Part model, mm, in its own coordinate system. A direction names the side the tool comes from. Give positions to 0.01 mm unless a question says otherwise; leave off trailing zeros. Loops run counter-clockwise (first coordinate to the right, second up) from the corner with the lowest first, then second, coordinate; pieces in that order, holes last. Notation, with made-up numbers: (34, 40) -> (40, 40) arc R21 cw to (40, 45) -> close; hole circle Ø1 at (31, -15). An arc over 180 degrees is marked (long way). One line per question, with ' | ' between items.
```python
from build123d import *

# Parameters (mm, degrees)
SKETCH1_W          = 42
SKETCH1_H          = 42
BASE_FLANGE1_DEPTH = 4
SKETCH4_R          = 2.25
TAB1_DEPTH         = 4
SKETCH5_R          = 12
SKETCH5_R_2        = 2
CUT_EXTRUDE1_DEPTH = 40.73977856


# Sheet-metal steps are written as plain solids
with BuildPart() as part:
    # Sketch1 → Base-Flange1 (new body)
    with BuildSketch(Plane(origin=(0, 0, 0), x_dir=(1, 0, 0), z_dir=(0, 1, 0))):
        Rectangle(SKETCH1_W, SKETCH1_H)
    extrude(amount=-BASE_FLANGE1_DEPTH)

    # Sketch4 → Tab1 (add)
    # profile 1 of 2: a face of its own
    with BuildSketch(Plane(origin=(0, 0, 0), x_dir=(1, 0, 0), z_dir=(0, 1, 0))):
        with BuildLine():
            Line((-9, 27.5), (-9, -27.5))
            ThreePointArc((-9, -27.5), (-15, -33.5), (-21, -27.5))
            Line((-21, -27.5), (-21, 27.5))
            ThreePointArc((-21, 27.5), (-15, 33.5), (-9, 27.5))
        make_face()
        with Locations(Location((-15, 27.5, 0), (0, 0, 270))):
            Circle(SKETCH4_R, mode=Mode.SUBTRACT)
        with Locations(Location((-15, -27.5, 0), (0, 0, 270))):
            Circle(SKETCH4_R, mode=Mode.SUBTRACT)
    # profile 2 of 2: a face of its own
    with BuildSketch(Plane(origin=(0, 0, 0), x_dir=(1, 0, 0), z_dir=(0, 1, 0))):
        with BuildLine():
            Line((21, 27.5), (21, -27.5))
            ThreePointArc((21, -27.5), (15, -33.5), (9, -27.5))
            Line((9, -27.5), (9, 27.5))
            ThreePointArc((9, 27.5), (15, 33.5), (21, 27.5))
        make_face()
        with Locations(Location((15, 27.5, 0), (0, 0, 270))):
            Circle(SKETCH4_R, mode=Mode.SUBTRACT)
        with Locations(Location((15, -27.5, 0), (0, 0, 270))):
            Circle(SKETCH4_R, mode=Mode.SUBTRACT)
    extrude(amount=-TAB1_DEPTH)

    # Sketch5 → Cut-Extrude1 (cut, through all)
    with BuildSketch(Plane(origin=(0, 0, 0), x_dir=(1, 0, 0), z_dir=(0, 1, 0))):
        with Locations(Location((0, 0, 0), (0, 0, 270))):
            Circle(SKETCH5_R)
        with Locations(Location((15.5, 15.5, 0), (0, 0, 270))):
            Circle(SKETCH5_R_2)
        with Locations(Location((15.5, -15.5, 0), (0, 0, 270))):
            Circle(SKETCH5_R_2)
        with Locations(Location((-15.5, -15.5, 0), (0, 0, 270))):
            Circle(SKETCH5_R_2)
        with Locations(Location((-15.5, 15.5, 0), (0, 0, 270))):
            Circle(SKETCH5_R_2)
    extrude(amount=-CUT_EXTRUDE1_DEPTH, mode=Mode.SUBTRACT)


solid = part.part
```
1) Saw through at B-B (x = 0). Give the cut face in (y, z).
Found:
outline: (-4, -21) -> (0, -21) -> (0, -12) -> (-4, -12) -> close; (-4, 12) -> (0, 12) -> (0, 21) -> (-4, 21) -> close
2) Tool access for faces 1 (the cylindrical face through (3.604, -1.972, 11.446)), 2 (the flat face through (-9, -2, -24)), 3 (the flat face through (0, -2, 21)): list every direction of +Z, -Z, +X, -X, +Y, -Y with a clear straight run to the whole face (end or side of a thin tool).
Found:
face 1: +Y, -Y | face 2: -Z, +Y, -Y | face 3: +Z, +Y, -Y
3) Saw through at D-D (y = -1.5). State how many separate pieces and enclosed holes the cut face has, and give its area (3 significant figures).
Found:
separate pieces: 1 | enclosed holes: 9 | area: 1,740 mm2
4) Pin check, flat tips, straight feed: P1, Ø2, axis at x = -5, y = -1, coming from the -Z side; P2, Ø1.2, axis at x = 0, y = -2, coming from the +Z side. Stop position of each tip, or through.
Found:
P1: z = -21 | P2: z = 21
5) Drill centre lines: line 1 (X direction, y = -2.3, z = 28.5); line 2 (Z direction, x = 16.5, y = -3); line 3 (X direction, y = -1, z = 14.5). Where is each one in solid material? Low to high.
Found:
line 1: -20.92 to -17.02, -12.98 to -9.08, 9.08 to 12.98, 17.02 to 20.92 | line 2: -33.31 to -29.18, -25.82 to -17.23, -13.77 to 13.77, 17.23 to 25.82, 29.18 to 33.31 | line 3: -21 to -17.23, -13.77 to 13.77, 17.23 to 21
6) Pull direction X, two halves, no side cores. Call faces 4 (the flat face through (10, 0, -8)), 5 (the cylindrical face through (-16.996, -1.972, -26.462)), 6 (the flat face through (-21, -2, 0)): pulls with the +X half, pulls with the -X half, needs draft (parallel to the pull), parting line crosses it, or undercut.
Found:
face 4: needs draft | face 5: undercut | face 6: pulls with the -X half
7) Saw through at C-C (z = 15.5). Give the cut face in (x, y).
Found:
outline: (-21, -4) -> (-17.5, -4) -> (-17.5, 0) -> (-21, 0) -> close; (-13.5, -4) -> (13.5, -4) -> (13.5, 0) -> (-13.5, 0) -> close; (17.5, -4) -> (21, -4) -> (21, 0) -> (17.5, 0) -> close
8) Saw through at A-A (z = 0). Give the cut face in (x, y), and give its area (3 significant figures).
Found:
outline: (-21, -4) -> (-12, -4) -> (-12, 0) -> (-21, 0) -> close; (12, -4) -> (21, -4) -> (21, 0) -> (12, 0) -> close | area: 72.0 mm2
